For this review, take the finished solid that the model builds, in its own axes (mm). Coordinates: 2 decimals unless noted, no trailing zeros. Loops run counter-clockwise (first coordinate to the right, second up) from the corner with the lowest first, then second, coordinate; pieces in that order, holes last. Notation, with made-up numbers: M 89.25,77.5 L 99.25,77.5 A24 cw 99.25,101.5 Z; hole C -14.5,57.25 d1. An arc over 180 degrees is marked long. Answer as a JSON object with one key per item and string values. Group by question number.
Item 1: Insertion check: pin 1 (3 mm diameter, centred on x = -15, z = 1.5, fed in from +Y); pin 2 (1.5 mm diameter, centred on x = 22.5, z = 2, fed in from -Y); pin 3 (6 mm diameter, centred on y = 0, z = 8, fed in from +X); pin 4 (1 mm diameter, centred on x = 23.5, z = 3.5, fed in from +Y). Each pin has a flat end and moves straight along its axis. Give the tip position at first contact, or say it passes through.
Item 2: Add section A-A (x = -1). State the section outline as (y, z) points.
Item 3: Add section B-B (y = -3). State the section outline as (x, z) points.
Item 4: Wall thickness on L1, parallel to Y at x = 12, z = 7.5; L2, parallel to X at y = 41.5, z = 5.25; L3, parallel to Y at x = 3, z = 7.25: over which ranges is each line inside the solid? List them lowest first. Write a range as from..to.
from build123d import *

# Parameters (mm, degrees)
F0_W     = 80
F0_H     = 100
F1_DEPTH = 10
F1_TAPER = 8
F2_R     = 10
F3_R     = 3


with BuildPart() as f1:
    # F0 (on Top) → F1 (new body)
    with BuildSketch(Plane.XY):
        Rectangle(F0_W, F0_H)
    extrude(amount=F1_DEPTH, taper=F1_TAPER)

    # F2
    f2_edges = [f1.edges().sort_by_distance(p)[0] for p in [
        (-39.297296, -49.297296, 5),
        (39.297296, -49.297296, 5),
        (39.297296, 49.297296, 5),
        (-39.297296, 49.297296, 5),
    ]]
    fillet(f2_edges, radius=F2_R)

    # F3
    f3_edges = [f1.edges().sort_by_distance(p)[0] for p in [
        (-38.594592, 0, 10),
    ]]
    fillet(f3_edges, radius=F3_R)


solid = f1.part
From the geometry:
{
 "1": {"pin 1": "stops at y = 50", "pin 2": "stops at y = -49.82", "pin 3": "stops at x = 39.3", "pin 4": "stops at y = 49.58"},
 "2": {"outline": "M -50,0 L 50,0 L 48.96,7.42 A3 ccw 45.99,10 L -45.99,10 A3 ccw -48.96,7.42 Z"},
 "3": {"outline": "M -40,0 L 40,0 L 38.96,7.42 A3 ccw 35.99,10 L -35.99,10 A3 ccw -38.96,7.42 Z"},
 "4": {"L1": "y = -48.94..48.94", "L2": "x = -39.03..39.03", "L3": "y = -48.98..48.98"}
}
